Source: CAD feature listing. Evaluate the final solid. Frame: model axes, mm. Give positions to 0.01 mm unless a question says otherwise; leave off trailing zeros. Order: outer loops, then holes, each group sorted by start corner. A loop starts at its lowest first (then second) coordinate and runs counter-clockwise, first axis right, second up. Notation, with made-up numbers: M 74,29 L 112,29 A19 cw 112,54 Z; hole C -10,-6 d7. An arc over 180 degrees is marked long. Use CSV: the item, a comma, the result in double quotes. Start each with the question number.
Item 1: Section query A-A on y = -58.5. Count the separate pieces of the cut face and the enclosed holes in it, and give its area (3 significant figures).
Item 2: Ray query, probe 1 along Y at (x, z) = (-71.5, 5); probe 2 along X at (y, z) = (53.5, 9); probe 3 along Y at (x, z) = (-72.5, 4.5). Return the intervals inside material, ascending. Write a range as from..to.
Item 3: Section query B-B on x = -112. Return loops of the section in (y, z), and give its area (3 significant figures).
Item 4: First-contact query: pin 1 (5 mm diameter, centred on y = -85.5, z = 3, fed in from -X); pin 2 (3 mm diameter, centred on x = -92, z = 7.5, fed in from +Y); pin 3 (3 mm diameter, centred on x = -72.5, y = 62, fed in from -Z); pin 4 (5 mm diameter, centred on y = -83.5, z = 7, fed in from +X). Flat tips, straight axial feed; report the tip coordinate or a pass-through.
Item 5: Section query C-C on y = 60.5. Return loops of the section in (x, z), and give its area (3 significant figures).
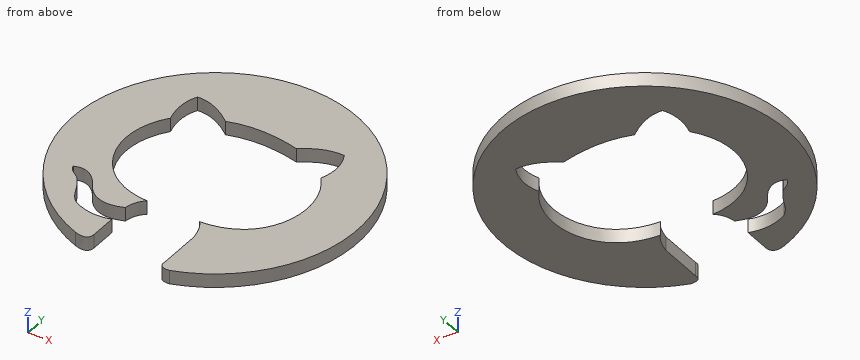
from build123d import *

# Parameters (mm, degrees)
RESSALTO_EXTRUS_O1_DEPTH = 10


with BuildPart() as part:
    # Esboço1 → Ressalto-extrusão1 (new body)
    with BuildSketch(Plane.XY):
        with BuildLine():
            Line((-7.232646643, -62.48429229), (-7.232646643, -94.533889528))
            add(Edge.make_bspline(
                [(0, -99.502819333), (-8.159285206, -100.402600429), (-7.232646643, -94.533889528)],
                knots=[0, 0, 0, 1, 1, 1], degree=2))
            ThreePointArc((0, -99.502819333), (-32.604573624, 102.237231854), (-69.037862067, -98.84663614))
            add(Edge.make_bspline(
                [(-69.037862067, -98.84663614), (-58.877940065, -102.146119369), (-58.412623628, -94.533889528)],
                knots=[0, 0, 0, 1, 1, 1], degree=2))
            Line((-58.412623628, -94.533889528), (-58.412623628, -75.403509781))
            add(Edge.make_bspline(
                [(-86.487077022, -72.670598389), (-72.514014981, -80.122898144), (-58.412623628, -75.403509781)],
                knots=[0, 0, 0, 1, 1, 1], degree=2))
            add(Edge.make_bspline(
                [(-100.648526965, -51.05575374), (-92.264568181, -60.681780492), (-93.93848024, -66.150620573), (-86.487077022, -72.670598389)],
                knots=[0, 0, 0, 0, 1, 1, 1, 1], degree=3))
            add(Edge.make_bspline(
                [(-108.350368162, -43.353912543), (-107.730240194, -46.867971027), (-104.99114076, -48.264073443), (-100.648526965, -51.05575374)],
                knots=[0, 0, 0, 0, 1, 1, 1, 1], degree=3))
            add(Edge.make_bspline(
                [(-86.487077022, -55.030897583), (-96.23915973, -38.074667842), (-108.350368162, -43.353912543)],
                knots=[0, 0, 0, 1, 1, 1], degree=2))
            add(Edge.make_bspline(
                [(-58.412623628, -60.993613349), (-76.239781836, -68.383433735), (-86.487077022, -55.030897583)],
                knots=[0, 0, 0, 1, 1, 1], degree=2))
            add(Edge.make_bspline(
                [(-51.456121902, -47.825949367), (-57.481841957, -52.926838867), (-58.412623628, -60.993613349)],
                knots=[0, 0, 0, 1, 1, 1], degree=2))
            add(Edge.make_bspline(
                [(-87.729309473, 30.434695052), (-112.261906541, -0.619225286), (-93.998220032, -46.894370576), (-51.456121902, -47.825949367)],
                knots=[0, 0, 0, 0, 1, 1, 1, 1], degree=3))
            add(Edge.make_bspline(
                [(-86.487077022, 57.515362486), (-92.384526984, 46.030854666), (-87.729309473, 30.434695052)],
                knots=[0, 0, 0, 1, 1, 1], degree=2))
            add(Edge.make_bspline(
                [(-58.412623628, 46.335270426), (-73.757926553, 58.757230824), (-86.487077022, 57.515362486)],
                knots=[0, 0, 0, 1, 1, 1], degree=2))
            add(Edge.make_bspline(
                [(-58.412623628, 46.335270426), (-36.364743942, 54.098608343), (-7.232646643, 47.080609896)],
                knots=[0, 0, 0, 1, 1, 1], degree=2))
            add(Edge.make_bspline(
                [(-7.232646643, 47.080609896), (6.307693164, 58.136478446), (20.593360262, 57.515362486)],
                knots=[0, 0, 0, 1, 1, 1], degree=2))
            add(Edge.make_bspline(
                [(20.593360262, 57.515362486), (27.4214118, 44.39924277), (21.835592713, 30.434695052)],
                knots=[0, 0, 0, 1, 1, 1], degree=2))
            add(Edge.make_bspline(
                [(21.835592713, 30.434695052), (43.574260816, 4.969398131), (33.44944429, -45.341538602), (-13.443808898, -47.825949367)],
                knots=[0, 0, 0, 0, 1, 1, 1, 1], degree=3))
            add(Edge.make_bspline(
                [(-13.443808898, -47.825949367), (-10.137665295, -50.925458995), (-8.474815726, -56.583989145), (-7.232646643, -62.48429229)],
                knots=[0, 0, 0, 0, 1, 1, 1, 1], degree=3))
        make_face()
    extrude(amount=RESSALTO_EXTRUS_O1_DEPTH)


solid = part.part
Verdict:
1,separate pieces,"3"
1,enclosed holes,"0"
1,area,"1,110 mm2"
2,probe 1,"-97.92..-77.16, -63.58..-43.48, 54.66..95.06"
2,probe 2,"-121.51..-88.18, -69.11..2.56, 22.39..54.33"
2,probe 3,"-97.52..-77.08, -63.5..-43.02, 55.09..94.66"
3,outline,"M -69.24,0 L 66.39,0 L 66.39,10 L -69.24,10 Z"
3,area,"1,360 mm2"
4,pin 1,"x = -97.57"
4,pin 2,"y = 85.22"
4,pin 3,"z = 0"
4,pin 4,"x = 32.86"
5,outline,"M -116.73,0 L 49.55,0 L 49.55,10 L -116.73,10 Z"
5,area,"1,660 mm2"
